Geometry check sheet. Reference: the model listing, model coordinates, mm. Round coordinates to 2 decimals unless told otherwise and drop trailing zeros. Order: outer loops, then holes, each group sorted by start corner. A loop starts at its lowest first (then second) coordinate and runs counter-clockwise, first axis right, second up.
(1) Sectioned sample at A-A (x = 0). Record the boundary of the cut face in (y, z), plus the area to 3 significant figures.
(2) Sectioned sample at C-C (y = 3). Record the boundary of the cut face in (x, z).
(3) Material ranges on line 1 along X through (y, z) = (22.5, 0.9); line 2 along Y through (x, z) = (33, 1.35); line 3 along X through (y, z) = (-3.5, 1.2), recorded low to high.
(4) Go/stop test with a flat-tipped pin: pin 1 (4.5 mm diameter, centred on x = 62.55, y = 25.11, fed in from -Z). Record where the tip stops, or that it passes through.
(5) Sectioned sample at D-D (x = 51). Record the boundary of the cut face in (y, z).
(6) Sectioned sample at B-B (z = 0.3). Record the boundary of the cut face in (x, y) (1 decimal), plus the area to 3 significant figures.
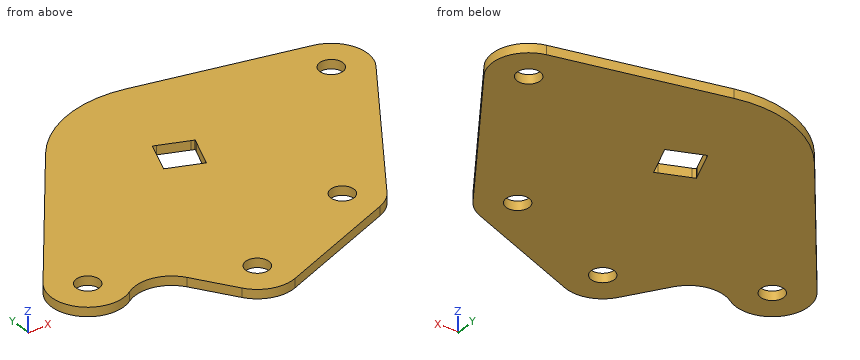
Autodesk Inventor part; units mm, degrees
ref_plane "YZ Plane" through (0, 0, 0) normal (1, 0, 0) x (0, 1, 0)
ref_plane "XZ Plane" through (0, 0, 0) normal (0, 1, 0) x (-1, 0, 0)
ref_plane "XY Plane" through (0, 0, 0) normal (0, 0, 1) x (1, 0, 0)
sketch "Sketch1" plane through (0, 0, 0) normal (0, 0, 1) x (1, 0, 0)
  circle A0 centre (0, 0) radius 2.0955 construction
  circle A1 centre (31.2825, 19.6012) radius 7.2 construction
  circle A2 centre (43.3748, -2.7357) radius 2.15 construction
  circle A3 centre (31.2825, 19.6012) radius 31.75 construction
  circle A4 centre (43.3748, -2.7357) radius 2.032
  line L0 (31.2825, 19.6012) -> (31.2825, -12.1488) construction
  circle A5 centre (31.2825, -12.1488) radius 2.032 construction
  line L1 (31.2825, 19.6012) -> (62.5502, 25.1146) construction
  line L2 (31.2825, 19.6012) -> (63.0325, 19.6012) construction
  circle A6 centre (62.5502, 25.1146) radius 2.032
  arc A7 (67.7804, 21.5135) -> (64.041, 31.2871) centre (62.5502, 25.1146) ccw
  circle A8 centre (0, 0) radius 2.032
  arc A9 (-5.017, 3.8926) -> (3.4439, -5.335) centre (0, 0) ccw
  arc A10 (45.62, -8.6755) -> (48.605, -6.3367) centre (43.3748, -2.7357) ccw
  circle A11 centre (22.0786, -10.7854) radius 2.032
  line L3 (48.605, -6.3367) -> (67.7804, 21.5135)
  arc A12 (35.755, 38.1188) -> (16.2316, 31.279) centre (31.2825, 19.6012) ccw
  line L4 (64.041, 31.2871) -> (35.755, 38.1188)
  line L5 (-5.017, 3.8926) -> (16.2316, 31.279)
  arc A13 (16.7437, -14.2294) -> (24.3239, -16.7253) centre (22.0786, -10.7854) ccw
  arc A14 (12.2228, -7.226) -> (3.4439, -5.335) centre (6.8878, -10.67) ccw
  line L6 (16.7437, -14.2294) -> (12.2228, -7.226)
  line L7 (45.9985, -8.5324) -> (24.3239, -16.7253)
  line L8 (27.7013, 17.6318) -> (32.3477, 15.7072)
  line L9 (27.7013, 17.6318) -> (27.7013, 17.6318)
  line L10 (32.3477, 15.7072) -> (27.7013, 17.6318)
  line L11 (32.3477, 15.7072) -> (32.3477, 15.7072)
  line L12 (33.1773, 16.0509) -> (35.1019, 20.6973)
  line L13 (33.1773, 16.0509) -> (33.1773, 16.0509)
  line L14 (35.1019, 20.6973) -> (33.1773, 16.0509)
  line L15 (35.1019, 20.6973) -> (35.1019, 20.6973)
  line L16 (34.7583, 21.5269) -> (30.1119, 23.4515)
  line L17 (34.7583, 21.5269) -> (34.7583, 21.5269)
  line L18 (30.1119, 23.4515) -> (34.7583, 21.5269)
  line L19 (30.1119, 23.4515) -> (30.1119, 23.4515)
  line L20 (29.2822, 23.1079) -> (27.3576, 18.4615)
  line L21 (29.2822, 23.1079) -> (29.2822, 23.1079)
  line L22 (27.3576, 18.4615) -> (29.2822, 23.1079)
  line L23 (27.3576, 18.4615) -> (27.3576, 18.4615)
  line L24 (35.1019, 20.6973) -> (35.3449, 21.2839)
  line L25 (34.7583, 21.5269) -> (35.3449, 21.2839)
  line L26 (33.1773, 16.0509) -> (32.9343, 15.4642)
  line L27 (32.3477, 15.7072) -> (32.9343, 15.4642)
  line L28 (29.2822, 23.1079) -> (29.5252, 23.6945)
  line L29 (30.1119, 23.4515) -> (29.5252, 23.6945)
  line L30 (27.3576, 18.4615) -> (27.1146, 17.8748)
  line L31 (27.7013, 17.6318) -> (27.1146, 17.8748)
  point P0 (0, 0)
extrude "Plate1" add sketch "Sketch1" along normal blind 1.5875
sketch "Sketch2" plane through (0, 0, 1.5875) normal (0, 0, 1) x (1, 0, 0)
  arc A0 (35.755, 38.1188) -> (16.2316, 31.279) centre (31.2825, 19.6012) ccw
  line L0 (35.755, 38.1188) -> (64.041, 31.2871)
  arc A1 (67.7804, 21.5135) -> (64.041, 31.2871) centre (62.5502, 25.1146) ccw
  line L1 (67.7804, 21.5135) -> (48.605, -6.3367)
  arc A2 (45.62, -8.6755) -> (48.605, -6.3367) centre (43.3748, -2.7357) ccw
  line L2 (45.62, -8.6755) -> (24.3239, -16.7253)
  arc A3 (16.7437, -14.2294) -> (24.3239, -16.7253) centre (22.0786, -10.7854) ccw
  line L3 (16.7437, -14.2294) -> (12.2228, -7.226)
  arc A4 (12.2228, -7.226) -> (3.4439, -5.335) centre (6.8878, -10.67) ccw
  arc A5 (-5.017, 3.8926) -> (3.4439, -5.335) centre (0, 0) ccw
  line L4 (-5.017, 3.8926) -> (16.2316, 31.279)
  circle A6 centre (0, 0) radius 2.032
  circle A7 centre (22.0786, -10.7854) radius 2.032
  circle A8 centre (43.3748, -2.7357) radius 2.032
  circle A9 centre (62.5502, 25.1146) radius 2.032
  line L5 (29.5252, 23.6945) -> (35.3449, 21.2839)
  line L6 (27.1146, 17.8748) -> (29.5252, 23.6945)
  line L7 (32.9343, 15.4642) -> (27.1146, 17.8748)
  line L8 (35.3449, 21.2839) -> (32.9343, 15.4642)
  point P0 (0, 0)
equation "\"d20\" = Thickness"
equation "\"BendRadius\" = Thickness"
equation "\"BendReliefWidth\" = Thickness"
equation "\"BendReliefDepth\" = 0.5 * Thickness"
equation "\"CornerReliefSize\" = 4 * Thickness"
equation "\"MinimumRemnant\" = 2 * Thickness"
equation "\"TransitionRadius\" = BendRadius"
equation "\"JacobiRadiusSize\" = BendRadius"
equation "\"GapSize\" = Thickness"
properties part number "Rear Vertical Odom Pod" material "Acetal Resin, White"
Answer below:
1. outline: (-6.35, 0) - (-2.03, 0) - (-2.03, 1.59) - (-6.35, 1.59) - close; (2.03, 0) - (10.36, 0) - (10.36, 1.59) - (2.03, 1.59) - close
1. area: 20.1 mm2
2. outline: (-5.6, 0) - (55.03, 0) - (55.03, 1.59) - (-5.6, 1.59) - close
3. line 1: x = 9.42 to 29.03, 32.41 to 68.34
3. line 2: y = -13.45 to 15.62, 22.26 to 38.57
3. line 3: x = -5.3 to 41.49, 45.26 to 50.56
4. pin 1: stops at z = 0
5. outline: (-2.86, 0) - (34.44, 0) - (34.44, 1.59) - (-2.86, 1.59) - close
6. outline: (-5, 3.9) arc R6.4 ccw to (3.4, -5.3) arc R6.3 cw to (12.2, -7.2) - (16.7, -14.2) arc R6.4 ccw to (24.3, -16.7) - (45.6, -8.7) arc R6.4 ccw to (48.6, -6.3) - (67.8, 21.5) arc R6.3 ccw to (64, 31.3) - (35.8, 38.1) arc R19 ccw to (16.2, 31.3) - close; hole circle Ø4.1 at (0, 0); hole circle Ø4.1 at (22.1, -10.8); hole (27.1, 17.9) - (27.7, 17.6) - (32.3, 15.7) - (32.9, 15.5) - (33.2, 16.1) - (35.1, 20.7) - (35.3, 21.3) - (34.8, 21.5) - (30.1, 23.5) - (29.5, 23.7) - (29.3, 23.1) - (27.4, 18.5) - close; hole circle Ø4.1 at (43.4, -2.7); hole circle Ø4.1 at (62.6, 25.1)
6. area: 2,520 mm2
